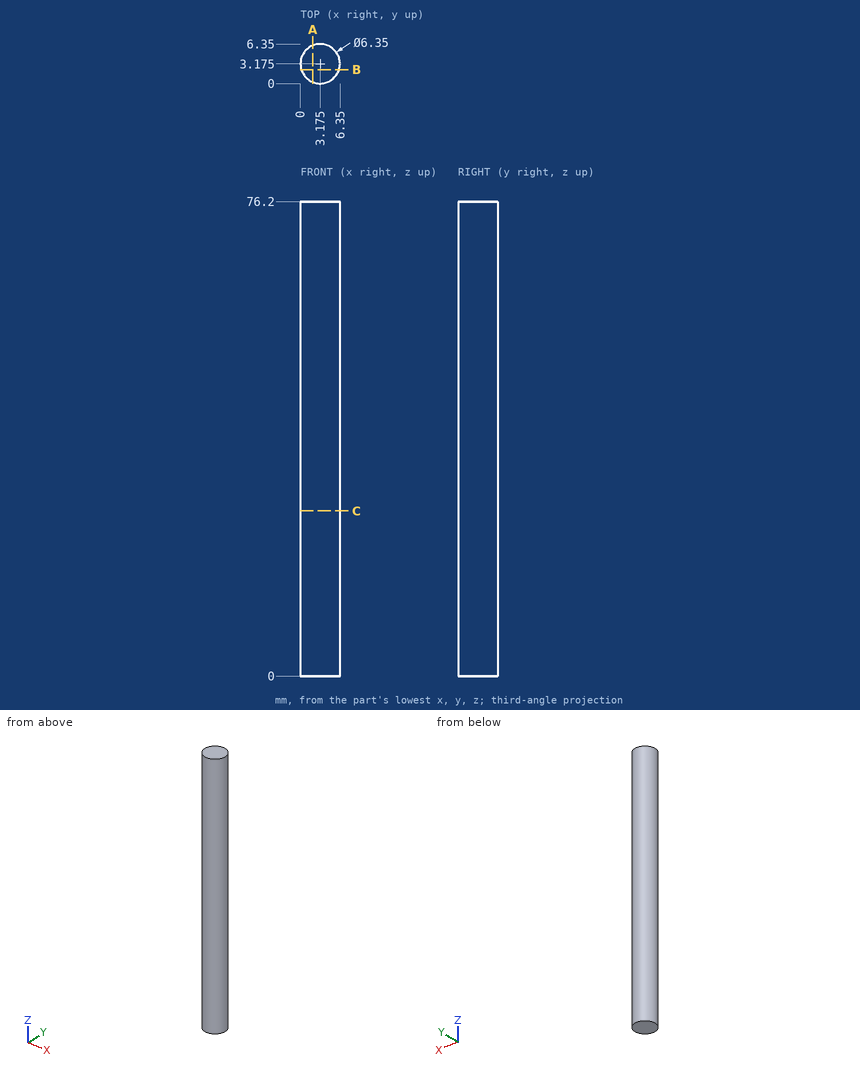
Verification items for this drawing (mm, ordinates from the low corner). Coordinates: 2 decimals unless noted, no trailing zeros. Order: outer loops, then holes, each group sorted by start corner. A loop starts at its lowest first (then second) coordinate and runs counter-clockwise, first axis right, second up. Notation, with made-up numbers: M 47,26 L 76,26 A25 ccw 76,65 Z; hole C -24.5,-9 d1. An arc over 180 degrees is marked long. One line per item, written item: value. Start each with the question number.
Item 1: Thickness scan on probe 1 along Y at (x, z) = (3, 24.5); probe 2 along Y at (x, z) = (0.5, 8); probe 3 along X at (y, z) = (1.5, 35). Record the ranges inside material, lowest first.
Item 2: Sectioned sample at C-C on z = 26.5. Record the cut outline in (x, y) (3 decimals), then the cut area to 3 significant figures.
Item 3: Sectioned sample at A-A on x = 2. Record the cut outline in (y, z), then the cut area to 3 significant figures.
Item 4: Sectioned sample at B-B on y = 2.25. Record the cut outline in (x, z), then the cut area to 3 significant figures.
Item 5: Depth check by flat-ended pin: P1, Ø2, axis at y = 1, z = 61, coming from the +X side. Enter the tip coordinate at first touch or a pass-through.
Calculated:
1. probe 1: 0 to 6.35
1. probe 2: 1.46 to 4.89
1. probe 3: 0.48 to 5.87
2. outline: C 3.175,3.175 d6.35
2. area: 31.7 mm^2
3. outline: M 0.23,0 L 6.12,0 L 6.12,76.2 L 0.23,76.2 Z
3. area: 450 mm^2
4. outline: M 0.14,0 L 6.21,0 L 6.21,76.2 L 0.14,76.2 Z
4. area: 463 mm^2
5. P1: x = 6.12
